The model under review builds one solid part; all positions refer to its coordinate system, in mm. A direction names the side the tool comes from. Give positions to 0.01 mm unless a question says otherwise; leave off trailing zeros. Order: outer loops, then holes, each group sorted by start corner. A loop starts at its lowest first (then second) coordinate and runs counter-clockwise, first axis right, second up. Notation, with made-up numbers: (89.5, 24) -> (106.5, 24) arc R28 ccw to (106.5, 44) -> close; hole circle Ø9 at (-3, -2). An arc over 180 degrees is marked (long way). Answer as a JSON object with one key per item and string values. Group by question number.
from build123d import *

# Parameters (mm, degrees)
CUT_EXTRUDE1_START = -4.064
SKETCH2_R          = 9.134112775
CUT_EXTRUDE1_DEPTH = 4.064


with BuildPart() as part:
    # Sketch1 → Revolve1 (revolve)
    with BuildSketch(Plane.XY):
        with BuildLine():
            Line((0, 1.5875), (11.1125, 1.5875))
            Line((11.1125, 1.5875), (11.1125, 4.882774376))
            Line((11.1125, 4.882774376), (21.2725, 5.1435))
            Line((21.2725, 5.1435), (21.2725, 6.699174823))
            Line((21.2725, 6.699174823), (25.3365, 6.699174823))
            Line((25.3365, 6.699174823), (25.3365, 1.5875))
            Line((25.3365, 1.5875), (28.426855679, 1.5875))
            Line((28.426855679, 1.5875), (28.426855679, 4.826))
            Line((28.426855679, 4.826), (85.7885, 4.826))
            Line((85.7885, 4.826), (85.7885, 0))
            Line((85.7885, 0), (0, 0))
            Line((0, 0), (-1.5875, 0))
            ThreePointArc((-1.5875, 0), (-1.122532015, 1.122532015), (0, 1.5875))
        make_face()
    revolve(axis=Axis((85.7885, 0, 0), (-1, 0, 0)))

    # Sketch2 → Cut-Extrude1 (cut)
    with BuildSketch(Plane(origin=(25.3365, 0, 0), x_dir=(0, 0, -1), z_dir=(1, 0, 0)).offset(CUT_EXTRUDE1_START)):
        Circle(SKETCH2_R)
        Polygon((6.699174823, 0), (3.349587412, 5.801655581), (-3.349587412, 5.801655581), (-6.699174823, 0), (-3.349587412, -5.801655581), (3.349587412, -5.801655581), align=None, mode=Mode.SUBTRACT)
    extrude(amount=CUT_EXTRUDE1_DEPTH, mode=Mode.SUBTRACT)


solid = part.part
1. Take a section at A-A on z = 0. Give the boundary of the cut face in (x, y) (1 decimal), plus the area to 3 significant figures.
2. For probe 1 along X at (y, z) = (-1.75, -1.75); probe 2 along Y at (x, z) = (66.5, 0); probe 3 along X at (y, z) = (-5, -1.5), list the stretches that pass through material, from the lowest coordinate up. Write a range as [from, to].
3. Take a section at C-C on x = 9. Give the boundary of the cut face in (y, z) (1 decimal).
4. Draft analysis for pull direction X (two halves, no side actions). For faces 1 (the flat face through (85.788, 0, 0)), 2 (the conical face through (16.26, -3.98, 3.05)), 3 (the flat face through (25.336, -1.4, 1.4)), 4 (the flat face through (23.28, 2.86, -5.05)), state which applies: pulls with the +X half, pulls with the -X half, needs draft (parallel to the pull), parting line crosses it, or undercut.
5. Machinability: for faces 5 (the flat face through (23, 5.802, 0)), 6 (the flat face through (28.427, 0, 2)), 7 (the flat face through (23, -5.802, 0)), 8 (the cylindrical face through (57.509, -3.83, 2.937)), 9 (the flat face through (11.112, 0, 2)), which of the approach directions +Z, -Z, +X, -X, +Y, -Y give a long, thin tool a straight path to every point of the face, cutting with its end or side? Answer none if there is none.
6. For pin 1 (2 mm diameter, centred on y = 1, z = -2, fed in from -X); pin 2 (1.5 mm diameter, centred on x = 55.5, y = 1, fed in from +Z); pin 3 (2 mm diameter, centred on x = 8, y = -3.5, fed in from +Z); pin 4 (3 mm diameter, centred on y = -2.5, z = -2, fed in from -X), all flat-tipped, find the tip position at first contact; note any pin that passes through.
7. Take a section at B-B on x = 63.5. Give the boundary of the cut face in (y, z).
Checks:
{
 "1": {"outline": "(0, -1.6) -> (11.1, -1.6) -> (11.1, -4.9) -> (21.3, -5.1) -> (21.3, -5.8) -> (25.3, -5.8) -> (25.3, -1.6) -> (28.4, -1.6) -> (28.4, -4.8) -> (85.8, -4.8) -> (85.8, 4.8) -> (28.4, 4.8) -> (28.4, 1.6) -> (25.3, 1.6) -> (25.3, 5.8) -> (21.3, 5.8) -> (21.3, 5.1) -> (11.1, 4.9) -> (11.1, 1.6) -> (0, 1.6) arc R1.6 ccw to start", "area": "752 mm2"},
 "2": {"probe 1": "x = [11.11, 25.34], [28.43, 85.79]", "probe 2": "y = [-4.83, 4.83]", "probe 3": "x = [21.27, 25.34]"},
 "3": {"outline": "circle Ø3.2 at (0, 0)"},
 "4": {"face 1": "pulls with the +X half", "face 2": "pulls with the -X half", "face 3": "undercut", "face 4": "needs draft"},
 "5": {"face 5": "+Z, -Z, +X, -X, +Y", "face 6": "none", "face 7": "+Z, -Z, +X, -X, -Y", "face 8": "+X", "face 9": "-X"},
 "6": {"pin 1": "stops at x = -1", "pin 2": "stops at z = 4.82", "pin 3": "passes through", "pin 4": "stops at x = 11.11"},
 "7": {"outline": "circle Ø9.65 at (0, 0)"}
}
